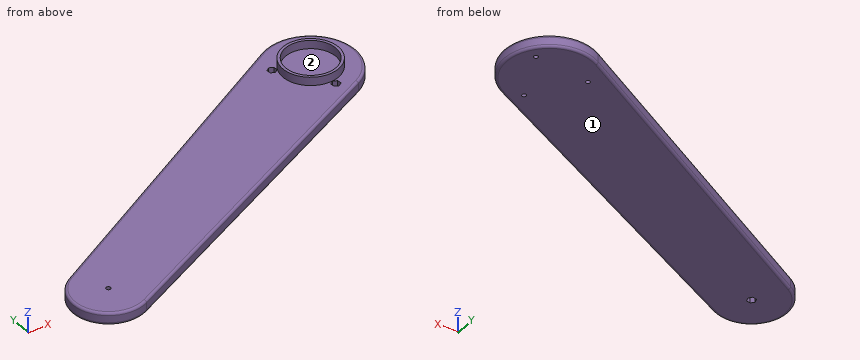
```python
from build123d import *

# Parameters (mm, degrees)
BOSS_EXTRUDE1_DEPTH = 10
FILLET1_R           = 2
SKETCH3_R           = 1.9
CUT_EXTRUDE3_DEPTH  = 240
CUT_EXTRUDE4_DEPTH  = 5
SKETCH6_R           = 1.75
CUT_EXTRUDE8_DEPTH  = 10
SKETCH7_R           = 23.25
SKETCH7_R_2         = 21
BOSS_EXTRUDE2_DEPTH = 7
CUT_EXTRUDE9_DEPTH  = 5


with BuildPart() as part:
    # Sketch1 → Boss-Extrude1 (new body)
    with BuildSketch(Plane.XY):
        with BuildLine():
            Line((-281.432373232, -110.20807274), (-17.900575614, 32.951773741))
            ThreePointArc((-17.900575614, 32.951773741), (33.388989093, 17.071186467), (16.23112616, -33.805333064))
            Line((16.23112616, -33.805333064), (-254.127011813, -163.613758184))
            ThreePointArc((-254.127011813, -163.613758184), (-293.823104015, -150.226440906), (-281.432373232, -110.20807274))
        make_face()
    extrude(amount=BOSS_EXTRUDE1_DEPTH)

    # Fillet1
    fillet1_edges = [part.edges().sort_by_distance(p)[0] for p in [
        (33.388989093, 17.071186467, 10),
        (-149.666474423, -38.628149499, 10),
        (-293.823104015, -150.226440906, 10),
        (-149.666474423, -38.628149499, 0),
        (33.388989093, 17.071186467, 0),
        (-118.947942827, -98.709545624, 0),
        (-293.823104015, -150.226440906, 0),
        (-118.947942827, -98.709545624, 10),
    ]]
    fillet(fillet1_edges, radius=FILLET1_R)

    # Sketch3 → Cut-Extrude3 (cut)
    with BuildSketch(Plane.XY.offset(10)):
        with Locations((-267.111912741, -136.569491732)):
            Circle(SKETCH3_R)
    extrude(amount=-CUT_EXTRUDE3_DEPTH, mode=Mode.SUBTRACT)

    # Sketch4 → Cut-Extrude4 (cut)
    with BuildSketch(Plane.XY.offset(10)):
        Polygon((1.949051074, -23.338757463), (-0.99159812, -25.380566053), (-0.693664608, -28.948147254), (2.544918098, -30.473919864), (5.485567292, -28.432111274), (5.18763378, -24.864530073), align=None)
        Polygon((19.237431318, 13.357306475), (22.476014024, 11.831533865), (25.416663218, 13.873342455), (25.118729706, 17.440923655), (21.880147001, 18.966696266), (18.939497807, 16.924887676), align=None)
        Polygon((-21.186482393, 9.981450988), (-21.484415905, 13.549032188), (-24.72299861, 15.074804799), (-27.663647804, 13.032996209), (-27.365714292, 9.465415008), (-24.127131587, 7.939642398), align=None)
    extrude(amount=-CUT_EXTRUDE4_DEPTH, mode=Mode.SUBTRACT)

    # Sketch6 → Cut-Extrude8 (cut)
    with BuildSketch(Plane.XY.offset(10)):
        with Locations((2.246984586, -26.906338663)):
            Circle(SKETCH6_R)
        with Locations((-24.425065098, 11.507223598)):
            Circle(SKETCH6_R)
        with Locations((22.178080512, 15.399115065)):
            Circle(SKETCH6_R)
    extrude(amount=-CUT_EXTRUDE8_DEPTH, mode=Mode.SUBTRACT)

    # Sketch7 → Boss-Extrude2 (add)
    with BuildSketch(Plane.XY.offset(10)):
        Circle(SKETCH7_R)
        Circle(SKETCH7_R_2, mode=Mode.SUBTRACT)
    extrude(amount=BOSS_EXTRUDE2_DEPTH)

    # Sketch8 → Cut-Extrude9 (cut)
    with BuildSketch(Plane(origin=(0, 0, 0), x_dir=(-1, 0, 0), z_dir=(0, 0, -1))):
        Polygon((270.635063904, -137.204948955), (269.42381042, -133.836081935), (265.900659257, -133.200624712), (263.588761578, -135.93403451), (264.800015061, -139.30290153), (268.323166224, -139.938358752), align=None)
    extrude(amount=-CUT_EXTRUDE9_DEPTH, mode=Mode.SUBTRACT)


solid = part.part
```
Part model, mm, in its own coordinate system. Face numbers are marked on the shaded views. Round coordinates to 2 decimals unless told otherwise and drop trailing zeros. Loops run counter-clockwise (first coordinate to the right, second up) from the corner with the lowest first, then second, coordinate; pieces in that order, holes last. Notation, with made-up numbers: (-8, 55) -> (49, 55) arc R26 cw to (49, 85) -> close; hole circle Ø5 at (74, 81.5). An arc over 180 degrees is marked (long way). Use CSV: the item, a comma, the result in double quotes. Start each with the question number.
1) Cut at A-A, the plane z = 13.25. Write the cut outline in (x, y), plus the area to 3 significant figures.
2) Pull direction Y, two halves, no side cores. Call the marked faces 1 and 2: +Y half, -Y half, draft (parallel to the pull), parting line (faces both ways), or undercut.
3) Wall check: L1, parallel to Y at x = 0, z = 14.5; L2, parallel to X at y = 3, z = 11.5; L3, parallel to X at y = -136, z = 6.5. Give the ranges that are in metal, low to high. Write a range as [from, to].
4) Drop flat-ended pins along their axis: P1, Ø4.5, axis at x = -267.11, y = -136.57, coming from the -Z side; P2, Ø1.9, axis at x = 3.5, y = -28.5, coming from the +Z side; P3, Ø8, axis at y = -77, z = 3, coming from the +X side; P4, Ø3, axis at x = 2.25, y = -26.91, coming from the +Z side. Give the stop position or say it passes through.
Determined:
1,outline,"circle Ø46.5 at (0, 0); hole circle Ø42 at (0, 0)"
1,area,"313 mm2"
2,face 1,"draft"
2,face 2,"undercut"
3,L1,"y = [-23.25, -21], [21, 23.25]"
3,L2,"x = [-23.06, -20.78], [20.78, 23.06]"
3,L3,"x = [-297.11, -268.92], [-265.3, -196.61]"
4,P1,"stops at z = 5"
4,P2,"stops at z = 5"
4,P3,"stops at x = -65.4"
4,P4,"passes through"
